Check sheet for the modelled part. Datum: model origin and axes. Units: mm. Give positions to 0.01 mm unless a question says otherwise; leave off trailing zeros. Order: outer loops, then holes, each group sorted by start corner. A loop starts at its lowest first (then second) coordinate and runs counter-clockwise, first axis right, second up.
```python
from build123d import *

# Parameters (mm, degrees)
SKETCH2_R           = 1.5
SKETCH2_W           = 74
SKETCH2_H           = 50.5
BOSS_EXTRUDE1_DEPTH = 2
SKETCH4_W           = 6
SKETCH4_H           = 60
BOSS_EXTRUDE3_DEPTH = 2
FILLET1_R           = 10


with BuildPart() as part:
    # Sketch2 → Boss-Extrude1 (new body)
    with BuildSketch(Plane(origin=(0, 0, 0), x_dir=(1, 0, 0), z_dir=(0, 1, 0))):
        with BuildLine():
            Line((-43.782705459, 34.194669068), (43.782705459, 34.194669068))
            ThreePointArc((43.782705459, 34.194669068), (55.303300859, 35.303300859), (54.194669068, 23.782705459))
            Line((54.194669068, 23.782705459), (54.194669068, -23.782705459))
            ThreePointArc((54.194669068, -23.782705459), (55.303300859, -35.303300859), (43.782705459, -34.194669068))
            Line((43.782705459, -34.194669068), (-43.782705459, -34.194669068))
            ThreePointArc((-43.782705459, -34.194669068), (-55.303300859, -35.303300859), (-54.194669068, -23.782705459))
            Line((-54.194669068, -23.782705459), (-54.194669068, 23.782705459))
            ThreePointArc((-54.194669068, 23.782705459), (-55.303300859, 35.303300859), (-43.782705459, 34.194669068))
        make_face()
        with Locations(Location((-50, -30, 0), (0, 0, 270))):
            Circle(SKETCH2_R, mode=Mode.SUBTRACT)
        with Locations(Location((50, -30, 0), (0, 0, 270))):
            Circle(SKETCH2_R, mode=Mode.SUBTRACT)
        with Locations(Location((-50, 30, 0), (0, 0, 270))):
            Circle(SKETCH2_R, mode=Mode.SUBTRACT)
        with Locations(Location((50, 30, 0), (0, 0, 270))):
            Circle(SKETCH2_R, mode=Mode.SUBTRACT)
        Rectangle(SKETCH2_W, SKETCH2_H, mode=Mode.SUBTRACT)
        with BuildLine():
            Line((51.5, 5.5), (51.5, -5.5))
            ThreePointArc((51.5, -5.5), (48, -9), (44.5, -5.5))
            Line((44.5, -5.5), (44.5, 5.5))
            ThreePointArc((44.5, 5.5), (48, 9), (51.5, 5.5))
        make_face(mode=Mode.SUBTRACT)
    extrude(amount=BOSS_EXTRUDE1_DEPTH)

    # Sketch4 → Boss-Extrude3 (add, through all)
    with BuildSketch(Plane(origin=(0, 2, 0), x_dir=(1, 0, 0), z_dir=(0, 1, 0))):
        with Locations((54.5, 0)):
            Rectangle(SKETCH4_W, SKETCH4_H)
    boss_extrude3 = extrude(amount=-BOSS_EXTRUDE3_DEPTH)

    # Mirror1: Boss-Extrude3 across plane
    add(boss_extrude3.mirror(Plane(origin=(0, 0, 0), x_dir=(0, 0, 1), z_dir=(1, 0, 0))))

    # Fillet1
    fillet1_edges = [part.edges().sort_by_distance(p)[0] for p in [
        (-43.782705459, 1, -34.194669068),
        (43.782705459, 1, -34.194669068),
        (43.782705459, 1, 34.194669068),
        (-43.782705459, 1, 34.194669068),
    ]]
    fillet(fillet1_edges, radius=FILLET1_R)


solid = part.part
```
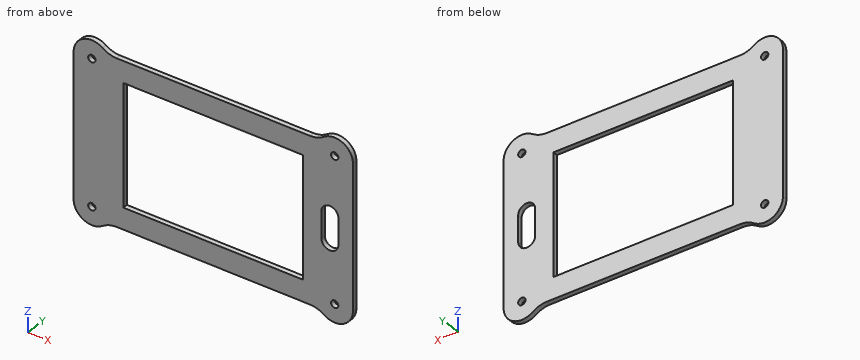
(1) Sectioned sample at D-D (x = -50). Enter the section's corners in (y, z).
(2) Thickness scan on L1, parallel to X at y = 1.2, z = -5.5; L2, parallel to X at y = 0.7, z = -30; L3, parallel to X at y = 1.7, z = 18.5. Record the ranges inside material, lowest first.
(3) Sectioned sample at B-B (x = -19). Enter the section's corners in (y, z).
(4) Go/stop test with flat-tipped pins: P1, Ø2.5, axis at x = 50, z = -30, coming from the -Y side; P2, Ø1, axis at x = -19.5, y = 0.5, coming from the -Z side; P3, Ø0.6, axis at x = -11, y = 1.5, coming from the +Z side. Record where each tip stops, or that it passes through.
(5) Sectioned sample at A-A (z = -20.5). Enter the section's corners in (x, y), plus the area to 3 significant figures.
(6) Sectioned sample at C-C (y = 0.85). Enter the section's corners in (x, z), plus the area to 3 significant figures.
Values follow:
1. outline: (0, -37.5) - (2, -37.5) - (2, -31.5) - (0, -31.5) - close; (0, -28.5) - (2, -28.5) - (2, 28.5) - (0, 28.5) - close; (0, 31.5) - (2, 31.5) - (2, 37.5) - (0, 37.5) - close
2. L1: x = -57.5 to -37, 37 to 44.5, 51.5 to 57.5
2. L2: x = -57.5 to -51.5, -48.5 to 48.5, 51.5 to 57.5
2. L3: x = -57.5 to -37, 37 to 57.5
3. outline: (0, -34.19) - (2, -34.19) - (2, -25.25) - (0, -25.25) - close; (0, 25.25) - (2, 25.25) - (2, 34.19) - (0, 34.19) - close
4. P1: passes through
4. P2: stops at z = -34.19
4. P3: stops at z = 34.19
5. outline: (-57.5, 0) - (-37, 0) - (-37, 2) - (-57.5, 2) - close; (37, 0) - (57.5, 0) - (57.5, 2) - (37, 2) - close
5. area: 82.0 mm2
6. outline: (-57.5, -30) arc R7.5 ccw to (-45.61, -36.08) arc R10 cw to (-39.76, -34.19) - (39.76, -34.19) arc R10 cw to (45.61, -36.08) arc R7.5 ccw to (57.5, -30) - (57.5, 30) arc R7.5 ccw to (45.61, 36.08) arc R10 cw to (39.76, 34.19) - (-39.76, 34.19) arc R10 cw to (-45.61, 36.08) arc R7.5 ccw to (-57.5, 30) - close; hole circle Ø3 at (-50, -30); hole circle Ø3 at (-50, 30); hole (-37, -25.25) - (37, -25.25) - (37, 25.25) - (-37, 25.25) - close; hole (44.5, -5.5) arc R3.5 ccw to (51.5, -5.5) - (51.5, 5.5) arc R3.5 ccw to (44.5, 5.5) - close; hole circle Ø3 at (50, -30); hole circle Ø3 at (50, 30)
6. area: 4,100 mm2
